```python
from build123d import *

# Parameters (mm, degrees)
SKETCH1_R          = 3.65
MAIN_EXTRUDE_DEPTH = 193.04


with BuildPart() as part:
    # Sketch1 → main Extrude (new body, symmetric)
    with BuildSketch(Plane(origin=(0, 0, 0), x_dir=(0, -1, 0), z_dir=(-1, 0, 0))):
        with BuildLine():
            Line((4.549996167, -15), (12.999943754, -15))
            Line((12.999943754, -15), (15, -12.999944234))
            Line((15, -12.999944234), (15, -4.54998765))
            ThreePointArc((15, -4.54998765), (14.853553391, -4.19643426), (14.5, -4.04998765))
            Line((14.5, -4.04998765), (13.299974565, -4.04998765))
            ThreePointArc((13.299974565, -4.04998765), (12.946421174, -4.19643426), (12.799974565, -4.54998765))
            Line((12.799974565, -4.54998765), (12.799974565, -8.249978163))
            Line((12.799974565, -8.249978163), (10.04886106, -8.249978163))
            Line((10.04886106, -8.249978163), (5.999989561, -4.201106482))
            Line((5.999989561, -4.201106482), (5.999989561, -0.899233628))
            Line((5.999989561, -0.899233628), (5.484990531, 5.429e-06))
            Line((5.484990531, 5.429e-06), (5.999989561, 0.899244177))
            Line((5.999989561, 0.899244177), (5.999989561, 4.232229952))
            Line((5.999989561, 4.232229952), (10.017749022, 8.249988862))
            Line((10.017749022, 8.249988862), (12.681560202, 8.249988862))
            Line((12.681560202, 8.249988862), (12.681560202, 4.549996167))
            ThreePointArc((12.681560202, 4.549996167), (12.828006812, 4.196442776), (13.181560202, 4.049996167))
            Line((13.181560202, 4.049996167), (14.5, 4.049996167))
            ThreePointArc((14.5, 4.049996167), (14.853553391, 4.196442776), (15, 4.549996167))
            Line((15, 4.549996167), (15, 12.999943159))
            Line((15, 12.999943159), (12.999943639, 15))
            Line((12.999943639, 15), (4.54998765, 15))
            ThreePointArc((4.54998765, 15), (4.19643426, 14.853553391), (4.04998765, 14.5))
            Line((4.04998765, 14.5), (4.04998765, 13.299974565))
            ThreePointArc((4.04998765, 13.299974565), (4.19643426, 12.946421174), (4.54998765, 12.799974565))
            Line((4.54998765, 12.799974565), (8.249978163, 12.799974565))
            Line((8.249978163, 12.799974565), (8.249978163, 10.04886106))
            Line((8.249978163, 10.04886106), (4.201106482, 5.999989561))
            Line((4.201106482, 5.999989561), (0.899233628, 5.999989561))
            Line((0.899233628, 5.999989561), (-5.358e-06, 5.484990655))
            Line((-5.358e-06, 5.484990655), (-0.899244177, 5.999989561))
            Line((-0.899244177, 5.999989561), (-4.232229952, 5.999989561))
            Line((-4.232229952, 5.999989561), (-8.249988862, 10.017749022))
            Line((-8.249988862, 10.017749022), (-8.249988862, 12.681560202))
            Line((-8.249988862, 12.681560202), (-4.549996167, 12.681560202))
            ThreePointArc((-4.549996167, 12.681560202), (-4.196442776, 12.828006812), (-4.049996167, 13.181560202))
            Line((-4.049996167, 13.181560202), (-4.049996167, 14.5))
            ThreePointArc((-4.049996167, 14.5), (-4.196442776, 14.853553391), (-4.549996167, 15))
            Line((-4.549996167, 15), (-12.999943355, 15))
            Line((-12.999943355, 15), (-15, 12.999943836))
            Line((-15, 12.999943836), (-15, 4.54998765))
            ThreePointArc((-15, 4.54998765), (-14.853553391, 4.19643426), (-14.5, 4.04998765))
            Line((-14.5, 4.04998765), (-13.299974565, 4.04998765))
            ThreePointArc((-13.299974565, 4.04998765), (-12.946421174, 4.19643426), (-12.799974565, 4.54998765))
            Line((-12.799974565, 4.54998765), (-12.799974565, 8.249978163))
            Line((-12.799974565, 8.249978163), (-10.048860846, 8.249978163))
            Line((-10.048860846, 8.249978163), (-5.999989347, 4.201106482))
            Line((-5.999989347, 4.201106482), (-5.999989347, 0.899233628))
            Line((-5.999989347, 0.899233628), (-5.484990531, -5.429e-06))
            Line((-5.484990531, -5.429e-06), (-5.999989347, -0.899244177))
            Line((-5.999989347, -0.899244177), (-5.999989347, -4.232229952))
            Line((-5.999989347, -4.232229952), (-10.017748808, -8.249988862))
            Line((-10.017748808, -8.249988862), (-12.681560202, -8.249988862))
            Line((-12.681560202, -8.249988862), (-12.681560202, -4.549996167))
            ThreePointArc((-12.681560202, -4.549996167), (-12.828006812, -4.196442776), (-13.181560202, -4.049996167))
            Line((-13.181560202, -4.049996167), (-14.5, -4.049996167))
            ThreePointArc((-14.5, -4.049996167), (-14.853553391, -4.196442776), (-15, -4.549996167))
            Line((-15, -4.549996167), (-15, -12.999948112))
            Line((-15, -12.999948112), (-12.999947631, -15))
            Line((-12.999947631, -15), (-4.54998765, -15))
            ThreePointArc((-4.54998765, -15), (-4.19643426, -14.853553391), (-4.04998765, -14.5))
            Line((-4.04998765, -14.5), (-4.04998765, -13.299974565))
            ThreePointArc((-4.04998765, -13.299974565), (-4.19643426, -12.946421174), (-4.54998765, -12.799974565))
            Line((-4.54998765, -12.799974565), (-8.249978163, -12.799974565))
            Line((-8.249978163, -12.799974565), (-8.249978163, -10.048860449))
            Line((-8.249978163, -10.048860449), (-4.201106482, -5.999988951))
            Line((-4.201106482, -5.999988951), (-0.899233628, -5.999988951))
            Line((-0.899233628, -5.999988951), (5.367e-06, -5.484990026))
            Line((5.367e-06, -5.484990026), (0.899244177, -5.999988951))
            Line((0.899244177, -5.999988951), (4.232229952, -5.999988951))
            Line((4.232229952, -5.999988951), (8.249988862, -10.017748412))
            Line((8.249988862, -10.017748412), (8.249988862, -12.681560202))
            Line((8.249988862, -12.681560202), (4.549996167, -12.681560202))
            ThreePointArc((4.549996167, -12.681560202), (4.196442776, -12.828006812), (4.049996167, -13.181560202))
            Line((4.049996167, -13.181560202), (4.049996167, -14.5))
            ThreePointArc((4.049996167, -14.5), (4.196442776, -14.853553391), (4.549996167, -15))
        make_face()
        Circle(SKETCH1_R, mode=Mode.SUBTRACT)
        with BuildLine():
            Line((-10.499978684, 9.499980695), (-12.6999746, 9.499980695))
            ThreePointArc((-12.6999746, 9.499980695), (-13.407079967, 9.792873328), (-13.6999726, 10.499978695))
            Line((-13.6999726, 10.499978695), (-13.6999726, 12.178655581))
            Line((-13.6999726, 12.178655581), (-12.178655571, 13.69997261))
            Line((-12.178655571, 13.69997261), (-10.499978695, 13.69997261))
            ThreePointArc((-10.499978695, 13.69997261), (-9.79287332, 13.407079974), (-9.499980684, 12.6999746))
            Line((-9.499980684, 12.6999746), (-9.499980684, 10.499978695))
            ThreePointArc((-9.499980684, 10.499978695), (-9.792873317, 9.792873328), (-10.499978684, 9.499980695))
        make_face(mode=Mode.SUBTRACT)
        with BuildLine():
            Line((9.499981, 10.499978695), (9.499981, 12.69997461))
            ThreePointArc((9.499981, 12.69997461), (9.792873633, 13.407079977), (10.499979, 13.69997261))
            Line((10.499979, 13.69997261), (12.178655581, 13.69997261))
            Line((12.178655581, 13.69997261), (13.69997261, 12.178655581))
            Line((13.69997261, 12.178655581), (13.69997261, 10.499978705))
            ThreePointArc((13.69997261, 10.499978705), (13.407079974, 9.792873331), (12.6999746, 9.499980695))
            Line((12.6999746, 9.499980695), (10.499979, 9.499980695))
            ThreePointArc((10.499979, 9.499980695), (9.792873633, 9.792873328), (9.499981, 10.499978695))
        make_face(mode=Mode.SUBTRACT)
        with BuildLine():
            Line((10.499979, -9.49998099), (12.69997461, -9.49998099))
            ThreePointArc((12.69997461, -9.49998099), (13.407079977, -9.792873623), (13.69997261, -10.49997899))
            Line((13.69997261, -10.49997899), (13.69997261, -12.178655571))
            Line((13.69997261, -12.178655571), (12.178655581, -13.6999726))
            Line((12.178655581, -13.6999726), (10.49997901, -13.6999726))
            ThreePointArc((10.49997901, -13.6999726), (9.792873636, -13.407079964), (9.499981, -12.69997459))
            Line((9.499981, -12.69997459), (9.499981, -10.49997899))
            ThreePointArc((9.499981, -10.49997899), (9.792873633, -9.792873623), (10.499979, -9.49998099))
        make_face(mode=Mode.SUBTRACT)
        with BuildLine():
            Line((-9.499980684, -10.49997899), (-9.499980684, -12.6999746))
            ThreePointArc((-9.499980684, -12.6999746), (-9.792873317, -13.407079967), (-10.499978684, -13.6999726))
            Line((-10.499978684, -13.6999726), (-12.178655571, -13.6999726))
            Line((-12.178655571, -13.6999726), (-13.6999726, -12.178655571))
            Line((-13.6999726, -12.178655571), (-13.6999726, -10.499979))
            ThreePointArc((-13.6999726, -10.499979), (-13.407079964, -9.792873626), (-12.69997459, -9.49998099))
            Line((-12.69997459, -9.49998099), (-10.499978684, -9.49998099))
            ThreePointArc((-10.499978684, -9.49998099), (-9.792873317, -9.792873623), (-9.499980684, -10.49997899))
        make_face(mode=Mode.SUBTRACT)
    extrude(amount=MAIN_EXTRUDE_DEPTH, both=True)


solid = part.part
```
The listing builds one solid part. Answer for the finished solid, in the listing's coordinates (mm). Round coordinates to 2 decimals unless told otherwise and drop trailing zeros. Use one line per item in the form item = value. Start each with the question number.
1. For a pull along Z with two mould halves and no side action, classify faces 1 (the face through (-3, -9, 15)), 2 (the face through (-3, -9, -15)), 3 (the face through (-3, 15, -9)), 4 (the face through (2.7, -3.48, 1.1)) as pulls with the +Z half, pulls with the -Z half, needs draft (parallel to the pull), parting line crosses it, or undercut.
2. Given pin 1 Ø5 at (x, z) = (0.5, 1.5) entering from +Y; pin 2 Ø10 at (y, z) = (7.5, -4.5) entering from -X; pin 3 Ø2.5 at (x, y) = (-5, -2.5) entering from -Z; pin 4 Ø1.7 at (x, z) = (-10, 3.5) entering from -Y, each flat-ended and moving along its own axis, determine where each tip first touches the part or whether it passes through.
3. Consider line 1 (Z direction, x = 83, y = -12.25); line 2 (Z direction, x = -149, y = 12.5); line 3 (Y direction, x = 41, z = 10.75). Determine where each line is inside the solid, lowest interval first. Write a range as [from, to].
4. The part is cut by section A-A on x = -158. Give the number of separate pieces and of enclosed holes in the cut face, then the cut area to 3 significant figures.
Geometry check:
q1.face_1 = pulls with the +Z half
q1.face_2 = pulls with the -Z half
q1.face_3 = needs draft
q1.face_4 = undercut
q2.pin_1 = 6
q2.pin_2 = -193.04
q2.pin_3 = -6
q2.pin_4 = -14.96
q3.line_1 = [-15, -13.63], [-9.5, -8.25], [8.25, 9.5], [13.63, 15]
q3.line_2 = [-15, -13.38], [-9.5, -8.25], [8.25, 9.5], [13.38, 15]
q3.line_3 = [-15, -13.7], [-9.5, -8.25], [8.25, 9.5], [13.7, 15]
q4.separate_pieces = 1
q4.enclosed_holes = 5
q4.area = 331 mm^2
